Here's how the part is built. I have some questions about the finished solid (model axes, mm). Face numbers are marked on the shaded views. A direction names the side the tool comes from. Coordinates: 2 decimals unless noted, no trailing zeros. Loops run counter-clockwise (first coordinate to the right, second up) from the corner with the lowest first, then second, coordinate; pieces in that order, holes last. Notation, with made-up numbers: (4, -11.75) -> (17, -11.75) arc R23 cw to (17, 12.25) -> close; hole circle Ø3 at (46, -38.5). An arc over 180 degrees is marked (long way). Answer as a JSON object with one key per item and string values. Group by question number.
Q1. On a 3-axis mill with a long thin cutter (end or side, diameter ignored), from which of +Z, -Z, +X, -X, +Y, -Y can I reach the whole of each face in a straight line? I mean the marked faces 5 and 6. Say none if no direction works.
Q2. I'm going to push a flat-ended pin straight in: pin 1 (10 mm diameter, centred on x = -68, z = 10, fed in from -Y). Where does the tip first touch, or does it pass through?
Q3. I need wall thicknesses on line 1 (X direction, y = 1, z = 10) (3 decimals); line 2 (Z direction, x = -10, y = 2); line 3 (Z direction, x = -28, y = 4.75). Which ranges of each line are inside material? Lowest first, please.
Q4. I want a section at C-C on z = 50. Write out the boundary of the cut face in (x, y) (3 decimals), then the cut area to 3 significant figures.
Q5. Thinking about a two-plate mould opening in Z: for the marked faces 1, 2, 3 and 4, which applies, released by +Z, released by -Z, zero draft, split by the parting line, or undercut?
Q6. I want a section at D-D on x = -39. Write out the boundary of the cut face in (y, z).
Q7. I want a section at A-A on x = -27. Write out the boundary of the cut face in (y, z), then the cut area to 4 significant figures.
Q8. I want a section at B-B on y = 5. Write out the boundary of the cut face in (x, z) (3 decimals), then the cut area to 3 significant figures.
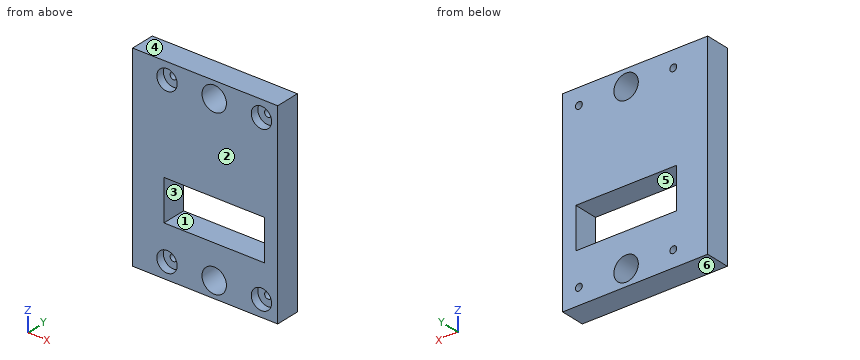
```python
from build123d import *

# Parameters (mm, degrees)
SKETCH1_W           = 89.125
SKETCH1_H           = 120
BOSS_EXTRUDE1_DEPTH = 7.5
CUT_EXTRUDE1_REACH  = 152.227
SKETCH3_W           = 61.75
SKETCH3_H           = 25
CUT_EXTRUDE2_REACH  = 152.227
SKETCH4_R           = 7.5
M5_TAPPED_HOLE1_D   = 4.2
SKETCH10_R          = 6.25
CUT_EXTRUDE3_DEPTH  = 5


with BuildPart() as part:
    # Sketch1 → Boss-Extrude1 (new, symmetric)
    with BuildSketch(Plane(origin=(0, 0, 0), x_dir=(1, 0, 0), z_dir=(0, 1, 0))):
        with Locations((-44.5625, -60)):
            Rectangle(SKETCH1_W, SKETCH1_H)
    extrude(amount=BOSS_EXTRUDE1_DEPTH, both=True)

    # Sketch3 → Cut-Extrude1 (cut, up to next)
    with BuildSketch(Plane(origin=(0, 7.5, 0), x_dir=(1, 0, 0), z_dir=(0, 1, 0)), mode=Mode.PRIVATE) as cut_extrude1_sk1:
        with Locations((-39, -43.22)):
            Rectangle(SKETCH3_W, SKETCH3_H)
    cut_extrude1_tool1 = extrude(cut_extrude1_sk1.sketch, amount=-CUT_EXTRUDE1_REACH, mode=Mode.PRIVATE) & part.part
    add(cut_extrude1_tool1.solids().sort_by_distance((-39, 7.5, 43.22))[0], mode=Mode.SUBTRACT)

    # Sketch4 → Cut-Extrude2 (cut, up to next)
    with BuildSketch(Plane(origin=(0, 7.5, 0), x_dir=(1, 0, 0), z_dir=(0, 1, 0)), mode=Mode.PRIVATE) as cut_extrude2_sk1:
        with Locations(Location((-39, -10, 0), (0, 0, 270))):
            Circle(SKETCH4_R)
    cut_extrude2_tool1 = extrude(cut_extrude2_sk1.sketch, amount=-CUT_EXTRUDE2_REACH, mode=Mode.PRIVATE) & part.part
    # Sketch4 → Cut-Extrude2 (cut, up to next)
    with BuildSketch(Plane(origin=(0, 7.5, 0), x_dir=(1, 0, 0), z_dir=(0, 1, 0)), mode=Mode.PRIVATE) as cut_extrude2_sk2:
        with Locations(Location((-39, -110, 0), (0, 0, 270))):
            Circle(SKETCH4_R)
    cut_extrude2_tool2 = extrude(cut_extrude2_sk2.sketch, amount=-CUT_EXTRUDE2_REACH, mode=Mode.PRIVATE) & part.part
    add(cut_extrude2_tool1.solids().sort_by_distance((-39, 7.5, 10))[0], mode=Mode.SUBTRACT)
    add(cut_extrude2_tool2.solids().sort_by_distance((-39, 7.5, 110))[0], mode=Mode.SUBTRACT)

    # M5 Tapped Hole1 (through all)
    with Locations(Plane(origin=(0, -7.5, 0), x_dir=(-1, 0, 0), z_dir=(0, -1, 0))):
        with Locations((10, -10), (68, -10), (68, -110), (10, -110)):
            Hole(M5_TAPPED_HOLE1_D / 2)

    # Sketch10 → Cut-Extrude3 (cut)
    with BuildSketch(Plane.XZ.offset(7.5)):
        with Locations(Location((-68, 110, 0), (0, 0, 270))):
            Circle(SKETCH10_R)
        with Locations(Location((-10, 110, 0), (0, 0, 270))):
            Circle(SKETCH10_R)
        with Locations(Location((-68, 10, 0), (0, 0, 270))):
            Circle(SKETCH10_R)
        with Locations(Location((-10, 10, 0), (0, 0, 270))):
            Circle(SKETCH10_R)
    extrude(amount=-CUT_EXTRUDE3_DEPTH, mode=Mode.SUBTRACT)


solid = part.part
```
Result set:
{
 "1": {"face 5": "+Y, -Y", "face 6": "-Z, +X, -X, +Y, -Y"},
 "2": {"pin 1": "stops at y = -2.5"},
 "3": {"line 1": "x = -89.125 to -70.1, -65.9 to -46.5, -31.5 to -12.1, -7.9 to 0", "line 2": "z = 0 to 7.9, 12.1 to 30.72, 55.72 to 107.9, 112.1 to 120", "line 3": "z = 0 to 30.72, 55.72 to 120"},
 "4": {"outline": "(-89.125, -7.5) -> (-69.875, -7.5) -> (-69.875, 7.5) -> (-89.125, 7.5) -> close; (-8.125, -7.5) -> (0, -7.5) -> (0, 7.5) -> (-8.125, 7.5) -> close", "area": "411 mm²"},
 "5": {"face 1": "undercut", "face 2": "zero draft", "face 3": "undercut", "face 4": "released by +Z"},
 "6": {"outline": "(-7.5, 0) -> (7.5, 0) -> (7.5, 2.5) -> (-7.5, 2.5) -> close; (-7.5, 17.5) -> (7.5, 17.5) -> (7.5, 30.72) -> (-7.5, 30.72) -> close; (-7.5, 55.72) -> (7.5, 55.72) -> (7.5, 102.5) -> (-7.5, 102.5) -> close; (-7.5, 117.5) -> (7.5, 117.5) -> (7.5, 120) -> (-7.5, 120) -> close"},
 "7": {"outline": "(-7.5, 0) -> (7.5, 0) -> (7.5, 30.72) -> (-7.5, 30.72) -> close; (-7.5, 55.72) -> (7.5, 55.72) -> (7.5, 120) -> (-7.5, 120) -> close", "area": "1,425 mm²"},
 "8": {"outline": "(-89.125, 0) -> (0, 0) -> (0, 120) -> (-89.125, 120) -> close; hole circle Ø4.2 at (-68, 10); hole circle Ø4.2 at (-68, 110); hole (-69.875, 30.72) -> (-8.125, 30.72) -> (-8.125, 55.72) -> (-69.875, 55.72) -> close; hole circle Ø15 at (-39, 10); hole circle Ø15 at (-39, 110); hole circle Ø4.2 at (-10, 10); hole circle Ø4.2 at (-10, 110)", "area": "8,740 mm²"}
}
